Verification items for the finished model (mm, model axes). Give positions to 0.01 mm unless a question says otherwise; leave off trailing zeros. Order: outer loops, then holes, each group sorted by start corner. A loop starts at its lowest first (then second) coordinate and runs counter-clockwise, first axis right, second up. Notation, with made-up numbers: (-28, 30) -> (-24, 30) arc R28 cw to (-24, 63) -> close; hole circle Ø11 at (70, -38). An arc over 180 degrees is marked (long way). Return JSON: item names as keys, results as strings. Group by question number.
(1) Thickness scan on line 1 along Z through (x, y) = (1.75, 24.5); line 2 along X through (y, z) = (13.25, 8); line 3 along X through (y, z) = (4.75, 3.25). Record the ranges inside material, lowest first.
(2) Cross-section at C-C on x = -6.5. Enter the section's corners in (y, z), then the cut area to 3 significant figures.
(3) Cross-section at B-B on z = -6.75. Enter the section's corners in (x, y).
(4) Depth check by flat-ended pin: pin 1 Ø3 at (y, z) = (15.5, -5) entering from -X; pin 2 Ø8 at (x, y) = (-7.5, 6.5) entering from -Z; pin 3 Ø4 at (x, y) = (3, 9.5) entering from +Z. Enter the tip coordinate at first touch or a pass-through.
(5) Cross-section at A-A on y = 14. Enter the section's corners in (x, z).
from build123d import *

# Parameters (mm, degrees)
SKETCH1_R           = 11
BOSS_EXTRUDE1_DEPTH = 27.94
SKETCH2_R           = 10.4267
CUT_EXTRUDE1_DEPTH  = 1.1684
SKETCH3_R           = 11
BOSS_EXTRUDE2_DEPTH = 20.32


with BuildPart() as part:
    # Sketch1 → Boss-Extrude1 (new body)
    with BuildSketch(Plane(origin=(0, 0, 0), x_dir=(1, 0, 0), z_dir=(0, 1, 0))):
        Circle(SKETCH1_R)
    extrude(amount=BOSS_EXTRUDE1_DEPTH)

    # Sketch2 → Cut-Extrude1 (cut)
    with BuildSketch(Plane(origin=(0, 12.954, 0), x_dir=(1, 0, 0), z_dir=(0, 1, 0))):
        with BuildLine():
            Line((-17.239436612, 14.563425366), (-16.28375247, -14.840830381))
            Line((-16.28375247, -14.840830381), (21.406068048, -16.295664576))
            Line((21.406068048, -16.295664576), (22.094276354, 14.197317514))
            Line((22.094276354, 14.197317514), (19.887741586, 14.563425366))
            ThreePointArc((19.887741586, 14.563425366), (1.324152487, 14.86501853), (-17.239436612, 14.563425366))
        make_face()
        Circle(SKETCH2_R, mode=Mode.SUBTRACT)
    extrude(amount=-CUT_EXTRUDE1_DEPTH, mode=Mode.SUBTRACT)

    # Sketch3 → Boss-Extrude2 (add)
    with BuildSketch(Plane.XZ):
        Circle(SKETCH3_R)
    extrude(amount=-BOSS_EXTRUDE2_DEPTH)


solid = part.part
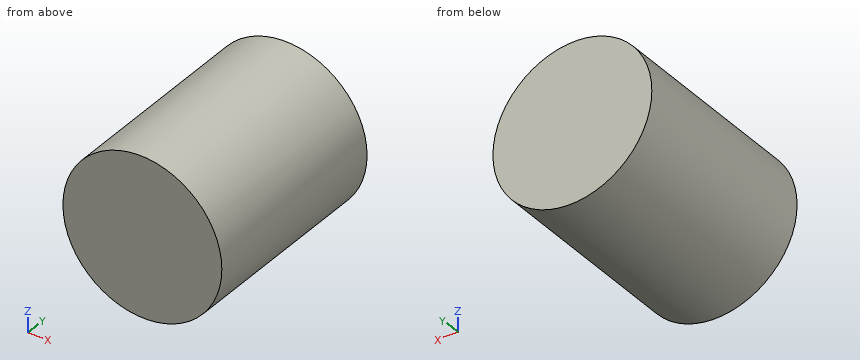
Verdict:
{
 "1": {"line 1": "-10.86 to 10.86", "line 2": "-7.55 to 7.55", "line 3": "-10.51 to 10.51"},
 "2": {"outline": "(0, -8.87) -> (27.94, -8.87) -> (27.94, 8.87) -> (0, 8.87) -> close", "area": "496 mm²"},
 "3": {"outline": "(-8.69, 0) -> (8.69, 0) -> (8.69, 27.94) -> (-8.69, 27.94) -> close"},
 "4": {"pin 1": "x = -10.43", "pin 2": "z = -10.43", "pin 3": "z = 10.95"},
 "5": {"outline": "circle Ø22 at (0, 0)"}
}
